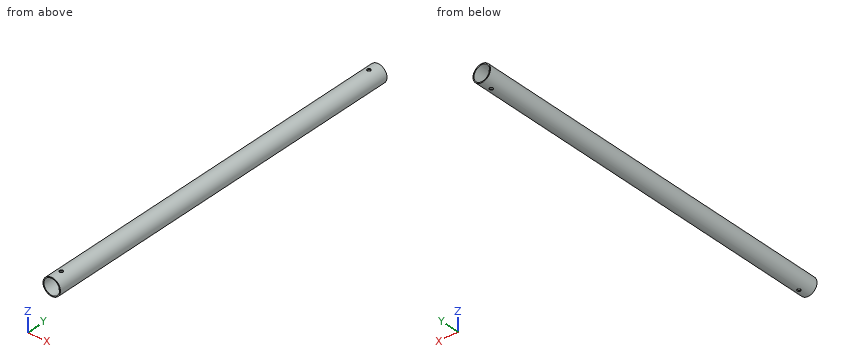
```python
from build123d import *

# Parameters (mm, degrees)
F0_R     = 24.15
F0_R_2   = 21.55
F1_DEPTH = 520
F4_D     = 10


with BuildPart() as f1:
    # F0 (on Front) → F1 (new body, symmetric)
    with BuildSketch(Plane.XZ):
        Circle(F0_R)
        Circle(F0_R_2, mode=Mode.SUBTRACT)
    extrude(amount=F1_DEPTH, both=True)

    # F4 (through all)
    with Locations(Plane.XY.offset(24.15)):
        with Locations((0, -490), (0, 490)):
            Hole(F4_D / 2)


solid = f1.part
```
The model under review builds one solid part; all positions refer to its coordinate system, in mm. Give positions to 0.01 mm unless a question says otherwise; leave off trailing zeros. Loops run counter-clockwise (first coordinate to the right, second up) from the corner with the lowest first, then second, coordinate; pieces in that order, holes last. Notation, with made-up numbers: (-28.75, 59.5) - (23.25, 59.5) arc R30 ccw to (23.25, 88.5) - close; hole circle Ø2 at (-20, 16.5). An arc over 180 degrees is marked (long way). Answer as a JSON object with one key per item and string values.
Q1. Add section A-A on x = -13. State the section outline as (y, z) points, plus the area to 3 significant figures.
Worked out:
{"outline": "(-520, -20.35) - (520, -20.35) - (520, -17.19) - (-520, -17.19) - close; (-520, 17.19) - (520, 17.19) - (520, 20.35) - (-520, 20.35) - close", "area": "6,580 mm^2"}
Q2. To check wall thickness, follow line 1 along Y through (x, z) = (0, 22); line 2 along Z through (x, y) = (0, 217); line 3 along X through (y, z) = (-385, 1.5). State the ranges of each line that lie inside material, in increasing order.
Worked out:
{"line 1": "y = -520 to -495, -485 to 485, 495 to 520", "line 2": "z = -24.15 to -21.55, 21.55 to 24.15", "line 3": "x = -24.1 to -21.5, 21.5 to 24.1"}
Q3. Add section B-B on z = -9. State the section outline as (x, y) points, plus the area to 3 significant figures.
Worked out:
{"outline": "(-22.41, -520) - (-19.58, -520) - (-19.58, 520) - (-22.41, 520) - close; (19.58, -520) - (22.41, -520) - (22.41, 520) - (19.58, 520) - close", "area": "5,890 mm^2"}
Q4. Add section C-C on y = 101.5. State the section outline as (x, z) points.
Worked out:
{"outline": "circle Ø48.3 at (0, 0); hole circle Ø43.1 at (0, 0)"}
Q5. Insertion check: pin 1 (2 mm diameter, centred on x = 2.5, y = -320, fed in from +Z); pin 2 (6 mm diameter, centred on y = 157.5, z = -16, fed in from +X). Each pin has a flat end and moves straight along its axis. Give the tip position at first contact, or say it passes through.
Worked out:
{"pin 1": "stops at z = 24.1", "pin 2": "stops at x = 20.35"}
